from build123d import *

# Parameters (mm, degrees)
SKETCH_1_R      = 1.6
SKETCH_1_W      = 6.1
SKETCH_1_H      = 10
EXTRUDE_1_DEPTH = 6


with BuildPart() as part:
    # Эскиз1 → Бобышка-Вытянуть1 (new body)
    with BuildSketch(Plane.XY):
        Polygon((1078.719864828, 623.038519), (1084.719864828, 623.138519), (1084.719864828, 633.138519), (1078.719864828, 633.238519), (1078.719864828, 723.038519), (1084.719864828, 723.138519), (1084.719864828, 733.138519), (1078.719864828, 733.238519), (1078.719864828, 761.588519), (1071.919864828, 761.588519), (1071.919864828, 760.388519), (1069.719864828, 760.388519), (1069.719864828, 761.588519), (1068.219864828, 761.588519), (1068.219864828, 764.688519), (1069.719864828, 764.688519), (1069.719864828, 765.888519), (1071.919864828, 765.888519), (1071.919864828, 764.688519), (1078.719864828, 764.688519), (1078.719864828, 793.038519), (1084.719864828, 793.138519), (1084.719864828, 803.138519), (1078.719864828, 803.238519), (1078.719864828, 836.338519), (978.719864828, 836.338519), (913.719864828, 836.338519), (913.719864828, 518.436195), (928.719864828, 518.436195), (928.719864828, 525.236195), (927.519864828, 525.236195), (927.519864828, 527.436195), (928.719864828, 527.436195), (928.719864828, 528.936195), (931.819864828, 528.936195), (931.819864828, 527.436195), (933.019864828, 527.436195), (933.019864828, 525.236195), (931.819864828, 525.236195), (931.819864828, 518.436195), (978.719864828, 518.436195), (1060.619864828, 518.436195), (1060.619864828, 525.236195), (1059.419864828, 525.236195), (1059.419864828, 527.436195), (1060.619864828, 527.436195), (1060.619864828, 528.936195), (1063.719864828, 528.936195), (1063.719864828, 527.436195), (1064.919864828, 527.436195), (1064.919864828, 525.236195), (1063.719864828, 525.236195), (1063.719864828, 518.436195), (1078.719864828, 518.436195), (1078.719864828, 553.038519), (1084.719864828, 553.138519), (1084.719864828, 563.138519), (1078.719864828, 563.238519), (1078.719864828, 591.588519), (1071.919864828, 591.588519), (1071.919864828, 590.388519), (1069.719864828, 590.388519), (1069.719864828, 591.588519), (1068.219864828, 591.588519), (1068.219864828, 594.688519), (1069.719864828, 594.688519), (1069.719864828, 595.888519), (1071.919864828, 595.888519), (1071.919864828, 594.688519), (1078.719864828, 594.688519), align=None)
        with Locations((919.269864828, 593.238519)):
            Circle(SKETCH_1_R, mode=Mode.SUBTRACT)
        with Locations((919.269864828, 763.238519)):
            Circle(SKETCH_1_R, mode=Mode.SUBTRACT)
        with Locations((975.719864828, 806.338519)):
            Circle(SKETCH_1_R, mode=Mode.SUBTRACT)
        with Locations((975.719864828, 674.138519)):
            Circle(SKETCH_1_R, mode=Mode.SUBTRACT)
        with Locations((975.719864828, 548.438519)):
            Circle(SKETCH_1_R, mode=Mode.SUBTRACT)
        with Locations((919.269864828, 558.238519)):
            Rectangle(SKETCH_1_W, SKETCH_1_H, mode=Mode.SUBTRACT)
        with Locations((919.269864828, 628.238519)):
            Rectangle(SKETCH_1_W, SKETCH_1_H, mode=Mode.SUBTRACT)
        with Locations((919.269864828, 728.238519)):
            Rectangle(SKETCH_1_W, SKETCH_1_H, mode=Mode.SUBTRACT)
        with Locations((919.269864828, 798.238519)):
            Rectangle(SKETCH_1_W, SKETCH_1_H, mode=Mode.SUBTRACT)
    extrude(amount=EXTRUDE_1_DEPTH)


solid = part.part
Check sheet for the modelled part. Datum: model origin and axes. Units: mm. A direction names the side the tool comes from. Round coordinates to 2 decimals unless told otherwise and drop trailing zeros. Loops run counter-clockwise (first coordinate to the right, second up) from the corner with the lowest first, then second, coordinate; pieces in that order, holes last. Notation, with made-up numbers: (-21, 60.25) -> (21, 60.25) arc R21 cw to (21, 91.25) -> close; hole circle Ø2 at (69.25, -12). An arc over 180 degrees is marked (long way). Put each result on its own line as item: value. Start each with the question number.
1. Section check B-B (y = 708.5). Enter the section's corners in (x, z).
2. Draft check along Y on faces 1 (the face through (916.22, 728, 3)), 2 (the face through (1063.72, 522, 3)), 3 (the face through (997, 836.339, 3)), 4 (the face through (922.32, 628, 3)). Enter one of: +Y half, -Y half, draft (parallel to the pull), parting line (faces both ways), or undercut.
3. Scan lines: probe 1 along Y at (x, z) = (1073.5, 5.7); probe 2 along X at (y, z) = (724.5, 2.7); probe 3 along X at (y, z) = (613, 1.1). Record each from-to range of solid material in increasing order.
4. Gauge pin test, flat end, axial feed: pin 1 (1.2 mm diameter, centred on y = 528, z = 4, fed in from +X). Record the tip position at first contact, or that the pin passes through.
5. Section check C-C (z = 0.9). Give the number of separate pieces and of enclosed holes in the cut face, plus the area to 3 significant figures.
6. Access from +Z, -Z, +X, -X, +Y, -Y to the whole of each face (thin tool, end or side, straight path). Record for faces 5 (the face through (928.72, 522, 3)), 6 (the face through (919, 803.239, 3)), 7 (the face through (1078.72, 535, 3)), 8 (the face through (1075, 761.589, 3)).
7. Section check A-A (y = 559). Enter the section's corners in (x, z).
Findings:
1. outline: (913.72, 0) -> (1078.72, 0) -> (1078.72, 6) -> (913.72, 6) -> close
2. face 1: undercut
2. face 2: draft
2. face 3: +Y half
2. face 4: undercut
3. probe 1: y = 518.44 to 591.59, 594.69 to 761.59, 764.69 to 836.34
3. probe 2: x = 913.72 to 916.22, 922.32 to 1084.72
3. probe 3: x = 913.72 to 1078.72
4. pin 1: stops at x = 1078.72
5. separate pieces: 1
5. enclosed holes: 9
5. area: 52,300 mm^2
6. face 5: +Z, -Z, -Y
6. face 6: +Z, -Z
6. face 7: +Z, -Z, +X, -Y
6. face 8: +Z, -Z, +X
7. outline: (913.72, 0) -> (916.22, 0) -> (916.22, 6) -> (913.72, 6) -> close; (922.32, 0) -> (1084.72, 0) -> (1084.72, 6) -> (922.32, 6) -> close
